Job drawing, mm, ordinate dimensions from the low corner. One solid piece. A direction names the side the tool comes from. Give positions to 0.01 mm unless a question says otherwise; leave off trailing zeros. Order: outer loops, then holes, each group sorted by start corner. A loop starts at its lowest first (then second) coordinate and runs counter-clockwise, first axis right, second up.
1. Slice it at C-C on z = 35.5. List the corners of the cut face in (x, y).
2. Slice it at A-A on x = 8.75. List the corners of the cut face in (y, z) (1 decimal), and give its area (3 significant figures).
3. Mould opens along X. For the marked faces 1, 2 and 3 say: +X half, -X half, draft (parallel to the pull), parting line (faces both ways), or undercut.
4. Which spindle directions (+Z, -Z, +X, -X, +Y, -Y) get a long thin tool onto all of the face, cutting with end or side? Do the marked faces 4 and 5. Say none if no direction does.
5. Drop flat-ended pins along their axis: pin 1 Ø1 at (x, z) = (13, 30) entering from +Y (1 decimal); pin 2 Ø1 at (y, z) = (13, 34) entering from -X; pin 3 Ø3 at (x, z) = (10, 20.5) entering from +Y (1 decimal). Give the stop position or say it passes through.
6. Probe line 1 (Z direction, x = 6.75, y = 7.5) (1 decimal); line 2 (X direction, y = 8, z = 39); line 3 (Z direction, x = 3, y = 2.25). List the from-to ranges inside material, lowest first.
7. Slice it at D-D on z = 4. List the corners of the cut face in (x, y) (1 decimal).
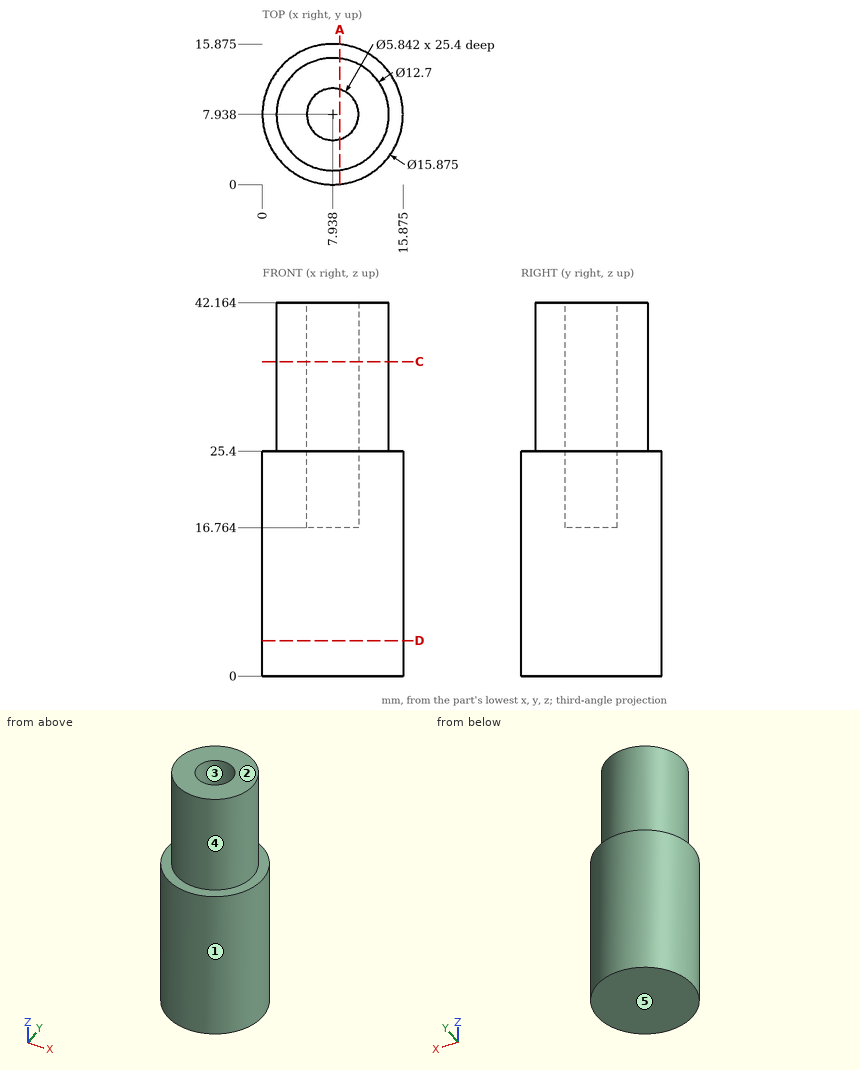
Data:
1. outline: circle Ø12.7 at (7.94, 7.94); hole circle Ø5.84 at (7.94, 7.94)
2. outline: (0, 0) - (15.8, 0) - (15.8, 25.4) - (14.2, 25.4) - (14.2, 42.2) - (10.7, 42.2) - (10.7, 16.8) - (5.1, 16.8) - (5.1, 42.2) - (1.6, 42.2) - (1.6, 25.4) - (0, 25.4) - close
2. area: 470 mm2
3. face 1: parting line
3. face 2: draft
3. face 3: undercut
4. face 4: +Z
4. face 5: -Z, +X, -X, +Y, -Y
5. pin 1: stops at y = 12.4
5. pin 2: stops at x = 3.52
5. pin 3: stops at y = 15.9
6. line 1: z = 0 to 16.8
6. line 2: x = 1.59 to 5.02, 10.86 to 14.29
6. line 3: z = 0 to 25.4
7. outline: circle Ø15.9 at (7.9, 7.9)
